Input: part model. Units: mm. Frame: model coordinates. A direction names the side the tool comes from. Coordinates: 2 decimals unless noted, no trailing zeros. Loops run counter-clockwise (first coordinate to the right, second up) from the corner with the lowest first, then second, coordinate; pieces in that order, holes last. Notation, with made-up numbers: (36.25, 19) -> (59.25, 19) arc R16 ccw to (59.25, 45) -> close; hole circle Ø1 at (27.25, 17). An arc over 180 degrees is marked (long way). Put each result on its own line as item: value. Start each with the question number.
1) Contact query for flat-ended pins moving along their axis: P1, Ø9, axis at x = -75, y = 30, coming from the -Z side; P2, Ø4.5, axis at x = 75, y = 0, coming from the +Z side; P3, Ø2, axis at x = 14, y = 1, coming from the +Z side; P4, Ø6, axis at x = 13.5, y = -33, coming from the -Z side. Output: stop coordinate, or through.
2) Cut plane B-B (z = 2.75). State how many separate pieces and enclosed holes the cut face has, plus the area to 3 significant figures.
3) Pull-direction query (Y, two-part tool) for faces 1 (the cylindrical face through (-29.97, 1.32, 4.44)), 2 (the flat face through (-1, -45, 6)); classes: pulls with the +Y half, pulls with the -Y half, needs draft (parallel to the pull), parting line crosses it, or undercut.
4) Material intervals for L1, parallel to Y at x = -7.75, z = 9.6; L2, parallel to X at y = -27.5, z = 1.75; L3, parallel to X at y = 1, z = 9.75, sorted ascending.
5) Cut plane A-A (x = 75). Return the cut outline in (y, z) (3 decimals).
6) Cut plane C-C (x = -15.5). Return the cut outline in (y, z).
7) Cut plane D-D (y = 38.5). Return the cut outline in (x, z).
8) Set-up query: faces 3 (the cylindrical face through (-79.87, 29.79, 2.46)), 4 (the cylindrical face through (77.747, -30.121, 8.549)), 5 (the cylindrical face through (7.05, 10.25, 10.52)). Return all of +Z, -Z, +X, -X, +Y, -Y with unobstructed straight access to the full face (end or side cutting, diameter ignored); none if empty.
from build123d import *

# Parameters (mm, degrees)
F0_W           = 180
F0_H           = 90
F0_R           = 42.5
F0_R_2         = 30
F1_DEPTH       = 12
F2_D           = 5.5
F2_CBORE_D     = 9.75
F2_CBORE_DEPTH = 5
F4_D           = 3.3
F4_CBORE_D     = 6.5
F4_CBORE_DEPTH = 3
F5_DEPTH       = 9


with BuildPart() as f1:
    # F0 (on Top) → F1 (new body)
    with BuildSketch(Plane.XY):
        Rectangle(F0_W, F0_H)
        Circle(F0_R, mode=Mode.SUBTRACT)
        Circle(F0_R)
        Circle(F0_R_2, mode=Mode.SUBTRACT)
        Circle(F0_R_2)
    extrude(amount=F1_DEPTH)

    # F2 (through all)
    with Locations(Plane(origin=(0, 0, 0), x_dir=(1, 0, 0), z_dir=(0, 0, -1))):
        with Locations((75, 30), (75, 0), (75, -30), (-75, -30), (-75, 0), (-75, 30)):
            CounterBoreHole(F2_D / 2, F2_CBORE_D / 2, F2_CBORE_DEPTH)

    # F4 (through all)
    with Locations(Plane.XY.offset(12)):
        with Locations((-15.5, 0), (-7.75, 13.4233937587), (7.75, 13.4233937587), (15.5, 0), (7.75, -13.4233937587), (-7.75, -13.4233937587)):
            CounterBoreHole(F4_D / 2, F4_CBORE_D / 2, F4_CBORE_DEPTH)

    # F0 (on Top) → F5 (cut)
    with BuildSketch(Plane.XY):
        Circle(F0_R)
        Circle(F0_R_2, mode=Mode.SUBTRACT)
    extrude(amount=F5_DEPTH, mode=Mode.SUBTRACT)


solid = f1.part
Results found:
1. P1: stops at z = 5
1. P2: passes through
1. P3: stops at z = 9
1. P4: stops at z = 9
2. separate pieces: 2
2. enclosed holes: 13
2. area: 12,900 mm2
3. face 1: undercut
3. face 2: pulls with the -Y half
4. L1: y = -45 to -16.67, -10.17 to 10.17, 16.67 to 45
4. L2: x = -90 to -79.19, -70.81 to -32.4, -11.99 to 11.99, 32.4 to 70.81, 79.19 to 90
4. L3: x = -90 to -77.56, -72.44 to -18.59, -12.41 to 12.41, 18.59 to 72.44, 77.56 to 90
5. outline: (-45, 0) -> (-34.875, 0) -> (-34.875, 5) -> (-32.75, 5) -> (-32.75, 12) -> (-45, 12) -> close; (-27.25, 5) -> (-25.125, 5) -> (-25.125, 0) -> (-4.875, 0) -> (-4.875, 5) -> (-2.75, 5) -> (-2.75, 12) -> (-27.25, 12) -> close; (2.75, 5) -> (4.875, 5) -> (4.875, 0) -> (25.125, 0) -> (25.125, 5) -> (27.25, 5) -> (27.25, 12) -> (2.75, 12) -> close; (32.75, 5) -> (34.875, 5) -> (34.875, 0) -> (45, 0) -> (45, 12) -> (32.75, 12) -> close
6. outline: (-45, 0) -> (-39.57, 0) -> (-39.57, 9) -> (-25.69, 9) -> (-25.69, 0) -> (-1.65, 0) -> (-1.65, 9) -> (-3.25, 9) -> (-3.25, 12) -> (-45, 12) -> close; (1.65, 0) -> (25.69, 0) -> (25.69, 9) -> (39.57, 9) -> (39.57, 0) -> (45, 0) -> (45, 12) -> (3.25, 12) -> (3.25, 9) -> (1.65, 9) -> close
7. outline: (-90, 0) -> (-18, 0) -> (-18, 9) -> (18, 9) -> (18, 0) -> (90, 0) -> (90, 12) -> (-90, 12) -> close
8. face 3: -Z
8. face 4: +Z, -Z
8. face 5: +Z
